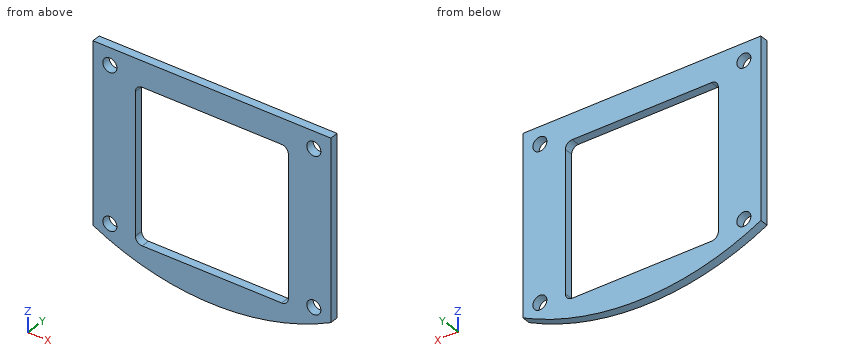
from build123d import *

# Parameters (mm, degrees)
SKETCH1_R           = 1.65
SKETCH1_W           = 36
SKETCH1_H           = 36
BOSS_EXTRUDE1_DEPTH = 2
FILLET1_R           = 1.6


with BuildPart() as part:
    # Sketch1 → Boss-Extrude1 (new body)
    with BuildSketch(Plane(origin=(0, 0, 0), x_dir=(1, 0, 0), z_dir=(0, 1, 0))):
        with BuildLine():
            Line((-28, -24), (28, -24))
            Line((28, -24), (28, 17.89570392))
            ThreePointArc((28, 17.89570392), (0, 24.701428863), (-28, 17.89570392))
            Line((-28, 17.89570392), (-28, -24))
        make_face()
        with Locations((-24, 16)):
            Circle(SKETCH1_R, mode=Mode.SUBTRACT)
        with Locations((-24, -20)):
            Circle(SKETCH1_R, mode=Mode.SUBTRACT)
        with Locations((24, 16)):
            Circle(SKETCH1_R, mode=Mode.SUBTRACT)
        with Locations((24, -20)):
            Circle(SKETCH1_R, mode=Mode.SUBTRACT)
        Rectangle(SKETCH1_W, SKETCH1_H, mode=Mode.SUBTRACT)
    extrude(amount=BOSS_EXTRUDE1_DEPTH)

    # Fillet1
    fillet1_edges = [part.edges().sort_by_distance(p)[0] for p in [
        (18, 1, -18),
        (-18, 1, -18),
        (-18, 1, 18),
        (18, 1, 18),
    ]]
    fillet(fillet1_edges, radius=FILLET1_R)


solid = part.part
The model under review builds one solid part; all positions refer to its coordinate system, in mm. Coordinates: 2 decimals unless noted, no trailing zeros. Write each loop counter-clockwise with the first axis right and the second up, starting at its lowest first coordinate (ties: lowest second). Pieces come first, ordered by that corner, then holes. Notation, with made-up numbers: (51.5, 49.25) - (102.5, 49.25) arc R25 cw to (102.5, 73.25) - close; hole circle Ø2 at (-37, 61). An arc over 180 degrees is marked (long way). Answer as a JSON object with one key per item and string values. Group by question number.
1. To check wall thickness, follow probe 1 along X at (y, z) = (1.55, -16); probe 2 along X at (y, z) = (1.7, -9); probe 3 along X at (y, z) = (1.5, 20). State the ranges of each line that lie inside material, in increasing order.
2. Add section A-A (z = 20). Give the boundary of the cut face in (x, y), plus the area to 3 significant figures.
3. Add section C-C (y = 0.9). Give the boundary of the cut face in (x, z), plus the area to 3 significant figures.
4. Add section D-D (x = -4.5). Give the boundary of the cut face in (y, z), plus the area to 3 significant figures.
5. Add section B-B (z = -7). Give the boundary of the cut face in (x, y).
Findings:
{
 "1": {"probe 1": "-28 to -25.65, -22.35 to -18, 18 to 22.35, 25.65 to 28", "probe 2": "-28 to -18, 18 to 28", "probe 3": "-28 to -25.65, -22.35 to 22.35, 25.65 to 28"},
 "2": {"outline": "(-28, 0) - (-25.65, 0) - (-25.65, 2) - (-28, 2) - close; (-22.35, 0) - (22.35, 0) - (22.35, 2) - (-22.35, 2) - close; (25.65, 0) - (28, 0) - (28, 2) - (25.65, 2) - close", "area": "98.8 mm²"},
 "3": {"outline": "(-28, -17.9) arc R61 ccw to (28, -17.9) - (28, 24) - (-28, 24) - close; hole circle Ø3.3 at (-24, -16); hole circle Ø3.3 at (-24, 20); hole (-18, -16.4) arc R1.6 ccw to (-16.4, -18) - (16.4, -18) arc R1.6 ccw to (18, -16.4) - (18, 16.4) arc R1.6 ccw to (16.4, 18) - (-16.4, 18) arc R1.6 ccw to (-18, 16.4) - close; hole circle Ø3.3 at (24, -16); hole circle Ø3.3 at (24, 20)", "area": "1,280 mm²"},
 "4": {"outline": "(0, -24.54) - (2, -24.54) - (2, -18) - (0, -18) - close; (0, 18) - (2, 18) - (2, 24) - (0, 24) - close", "area": "25.1 mm²"},
 "5": {"outline": "(-28, 0) - (-18, 0) - (-18, 2) - (-28, 2) - close; (18, 0) - (28, 0) - (28, 2) - (18, 2) - close"}
}
